from build123d import *

# Parameters (mm, degrees)
F0_R     = 15
F1_DEPTH = 30
F2_DEPTH = 24
F3_W     = 406
F3_H     = 725
F3_R     = 15
F4_DEPTH = 4


# Not quite as in the source:
# - a feature names something its author has since deleted; it is built from what else it names


with BuildPart() as f1:
    # F0 (on Top) → F1 (new body)
    with BuildSketch(Plane.XY):
        with BuildLine():
            ThreePointArc((4355.1985619355, -294.5215593797), (4377.1655533465, -347.5545679687), (4430.1985619355, -369.5215593797))
            Line((4430.1985619355, -369.5215593797), (4753.0624461818, -369.5215593797))
            ThreePointArc((4753.0624461818, -369.5215593797), (5255.1985619355, -332.6549530029), (5757.3346776893, -369.5215593797))
            Line((5757.3346776893, -369.5215593797), (6080.1985619355, -369.5215593797))
            ThreePointArc((6080.1985619355, -369.5215593797), (6133.2315705245, -347.5545679687), (6155.1985619355, -294.5215593797))
            Line((6155.1985619355, -294.5215593797), (6155.1985619355, 430.4784406203))
            Line((6155.1985619355, 430.4784406203), (4355.1985619355, 430.4784406203))
            Line((4355.1985619355, 430.4784406203), (4355.1985619355, -294.5215593797))
        make_face()
        with BuildLine():
            Line((6065.1985619355, 163.3609871071), (6065.1985619355, -195.1546647585))
            Line((6065.1985619355, -195.1546647585), (6065.1985619355, -204.4389326959))
            Line((6065.1985619355, -204.4389326959), (6065.1159855294, -205.7217836249))
            ThreePointArc((6065.1159855294, -205.7217836249), (6040.8429178387, -255.0832383215), (5991.4814631421, -279.3563060122))
            Line((5991.4814631421, -279.3563060122), (5990.1985619355, -279.5026946765))
            Line((5990.1985619355, -279.5026946765), (5968.0089636665, -279.5215593797))
            Line((5968.0089636665, -279.5215593797), (5745.1985619355, -279.5215593797))
            Line((5745.1985619355, -279.5215593797), (5745.1985619355, 102.1975441552))
            Line((5745.1985619355, 102.1975441552), (5745.2811886192, 146.843918233))
            ThreePointArc((5745.2811886192, 146.843918233), (5769.55425631, 196.2053729296), (5818.9157110066, 220.4784406203))
            Line((5818.9157110066, 220.4784406203), (6065.1985619355, 220.4784406203))
            Line((6065.1985619355, 220.4784406203), (6065.1985619355, 163.3609871071))
        make_face(mode=Mode.SUBTRACT)
        with Locations((4505.1985619355, 310.4784406203)):
            Circle(F0_R, mode=Mode.SUBTRACT)
        with Locations((6005.1985619355, 310.4784406203)):
            Circle(F0_R, mode=Mode.SUBTRACT)
    extrude(amount=F1_DEPTH)

    # F0 (on Top) → F2 (join)
    with BuildSketch(Plane.XY):
        with BuildLine():
            Line((6065.1985619355, -204.4389326959), (6065.1985619355, -195.1546647585))
            Line((6065.1985619355, -195.1546647585), (6065.1985619355, 163.3609871071))
            Line((6065.1985619355, 163.3609871071), (6065.1985619355, 220.4784406203))
            Line((6065.1985619355, 220.4784406203), (5818.9157110066, 220.4784406203))
            ThreePointArc((5818.9157110066, 220.4784406203), (5769.55425631, 196.2053729296), (5745.2811886192, 146.843918233))
            Line((5745.2811886192, 146.843918233), (5745.1985619355, 102.1975441552))
            Line((5745.1985619355, 102.1975441552), (5745.1985619355, -279.5215593797))
            Line((5745.1985619355, -279.5215593797), (5968.0089636665, -279.5215593797))
            Line((5968.0089636665, -279.5215593797), (5990.1985619355, -279.5026946765))
            Line((5990.1985619355, -279.5026946765), (5991.4814631421, -279.3563060122))
            ThreePointArc((5991.4814631421, -279.3563060122), (6040.8429178387, -255.0832383215), (6065.1159855294, -205.7217836249))
            Line((6065.1159855294, -205.7217836249), (6065.1985619355, -204.4389326959))
        make_face()
    extrude(amount=F2_DEPTH)

    # F3 (on face) + F0 (on Top) → F4 (cut)
    with BuildSketch(Plane.XY):
        with Locations((5902.1985619355, 57.9784406203)):
            Rectangle(F3_W, F3_H)
        with BuildLine():
            Line((6065.1985619355, 220.4784406203), (6065.1985619355, 163.3609871071))
            Line((6065.1985619355, 163.3609871071), (6065.1985619355, -195.1546647585))
            Line((6065.1985619355, -195.1546647585), (6065.1985619355, -204.4389326959))
            Line((6065.1985619355, -204.4389326959), (6065.1159855294, -205.7217836249))
            ThreePointArc((6065.1159855294, -205.7217836249), (6040.8429178387, -255.0832383215), (5991.4814631421, -279.3563060122))
            Line((5991.4814631421, -279.3563060122), (5990.1985619355, -279.5026946765))
            Line((5990.1985619355, -279.5026946765), (5968.0089636665, -279.5215593797))
            Line((5968.0089636665, -279.5215593797), (5745.1985619355, -279.5215593797))
            Line((5745.1985619355, -279.5215593797), (5745.1985619355, 102.1975441552))
            Line((5745.1985619355, 102.1975441552), (5745.2811886192, 146.843918233))
            ThreePointArc((5745.2811886192, 146.843918233), (5769.55425631, 196.2053729296), (5818.9157110066, 220.4784406203))
            Line((5818.9157110066, 220.4784406203), (6065.1985619355, 220.4784406203))
        make_face(mode=Mode.SUBTRACT)
        with Locations((6005.1985619355, 310.4784406203)):
            Circle(F3_R, mode=Mode.SUBTRACT)
    with BuildSketch(Plane.XY):
        with BuildLine():
            Line((6065.1985619355, -204.4389326959), (6065.1985619355, -195.1546647585))
            Line((6065.1985619355, -195.1546647585), (6065.1985619355, 163.3609871071))
            Line((6065.1985619355, 163.3609871071), (6065.1985619355, 220.4784406203))
            Line((6065.1985619355, 220.4784406203), (5818.9157110066, 220.4784406203))
            ThreePointArc((5818.9157110066, 220.4784406203), (5769.55425631, 196.2053729296), (5745.2811886192, 146.843918233))
            Line((5745.2811886192, 146.843918233), (5745.1985619355, 102.1975441552))
            Line((5745.1985619355, 102.1975441552), (5745.1985619355, -279.5215593797))
            Line((5745.1985619355, -279.5215593797), (5968.0089636665, -279.5215593797))
            Line((5968.0089636665, -279.5215593797), (5990.1985619355, -279.5026946765))
            Line((5990.1985619355, -279.5026946765), (5991.4814631421, -279.3563060122))
            ThreePointArc((5991.4814631421, -279.3563060122), (6040.8429178387, -255.0832383215), (6065.1159855294, -205.7217836249))
            Line((6065.1159855294, -205.7217836249), (6065.1985619355, -204.4389326959))
        make_face()
    extrude(amount=F4_DEPTH, mode=Mode.SUBTRACT)


solid = f1.part
Could you check a few things on this model? Use its own coordinates, in mm. A direction names the side the tool comes from. Give positions to 0.01 mm unless a question says otherwise; leave off trailing zeros. Loops run counter-clockwise (first coordinate to the right, second up) from the corner with the lowest first, then second, coordinate; pieces in that order, holes last. Notation, with made-up numbers: M 57,-20.75 L 62,-20.75 A15 cw 62,-4.75 Z; hole C 76,8 d2. An arc over 180 degrees is marked long. Answer as a JSON object with one key per item and string values.
Q1. Suppose I cut it at A-A, the plane y = -140.5. List the corners of the cut face in (x, z) for me.
Values found:
{"outline": "M 4355.2,0 L 5699.2,0 L 5699.2,4 L 6105.2,4 L 6105.2,0 L 6155.2,0 L 6155.2,30 L 6065.2,30 L 6065.2,24 L 5745.2,24 L 5745.2,30 L 4355.2,30 Z"}
Q2. Suppose I cut it at D-D, the plane x = 5425. List the corners of the cut face in (y, z) for me, plus the area to 3 significant figures.
Values found:
{"outline": "M -336.85,0 L 430.48,0 L 430.48,30 L -336.85,30 Z", "area": "23,000 mm²"}
Q3. For faces 4 (the flat face through (5268, 430.478, 15)), 5 (the flat face through (5899, 63, 4)), 6 (the cylindrical face through (5769.002, 195.648, 26.958)), which set-ups out of +Z, -Z, +X, -X, +Y, -Y let a thin tool reach every point of the face, with its end or its side?
Values found:
{"face 4": "+Z, -Z, +X, -X, +Y", "face 5": "-Z", "face 6": "+Z"}
Q4. If I drill on probe 1 along X at (y, z) = (-62, 28.5); probe 2 along Z at (x, y) = (5905, 332); probe 3 along Z at (x, y) = (5924, -167), over which ranges is the centre line in solid material (lowest first)? Write a range as [from, to].
Values found:
{"probe 1": "x = [4355.2, 5745.2], [6065.2, 6155.2]", "probe 2": "z = [4, 30]", "probe 3": "z = [4, 24]"}
Q5. If we mould it in two halves opening along X, with no side actions, what happens to faces 1 (the cylindrical face through (6132.65, -348.13, 14.79)), 2 (the flat face through (4589, -369.522, 15)), 3 (the cylindrical face through (4519.5, 315, 14.8))? For each: pulls with the +X half, pulls with the -X half, needs draft (parallel to the pull), parting line crosses it, or undercut.
Values found:
{"face 1": "pulls with the +X half", "face 2": "needs draft", "face 3": "undercut"}
Q6. Suppose I cut it at C-C, the plane y = 279. List the corners of the cut face in (x, z) for me.
Values found:
{"outline": "M 4355.2,0 L 5699.2,0 L 5699.2,4 L 6105.2,4 L 6105.2,0 L 6155.2,0 L 6155.2,30 L 4355.2,30 Z"}
Q7. Suppose I cut it at B-B, the plane z = 17.5. List the corners of the cut face in (x, y) for me.
Values found:
{"outline": "M 4355.2,-294.52 A75 ccw 4430.2,-369.52 L 4753.06,-369.52 A3438.07 cw 5757.33,-369.52 L 6080.2,-369.52 A75 ccw 6155.2,-294.52 L 6155.2,430.48 L 4355.2,430.48 Z; hole C 4505.2,310.48 d30; hole C 6005.2,310.48 d30"}
